```python
from build123d import *

# Parameters (mm, degrees)
BOSS_EXTRUDE1_DEPTH = 2
CUT_EXTRUDE1_REACH  = 137.359
SKETCH2_W           = 110
SKETCH2_H           = 10
SKETCH3_W           = 15
SKETCH3_H           = 4
BOSS_EXTRUDE2_DEPTH = 4


with BuildPart() as part:
    # Sketch1 → Boss-Extrude1 (new, symmetric)
    with BuildSketch(Plane.XY):
        Polygon((-105, -5), (-75, -5), (-75, -9), (-45, -9), (-45, -5), (-15, -5), (-15, -9), (15, -9), (15, -5), (45, -5), (45, -9), (75, -9), (75, -5), (105, -5), (105, -9), (135, -9), (135, -5), (135, 5), (135, 9), (105, 9), (105, 5), (75, 5), (75, 9), (45, 9), (45, 5), (15, 5), (15, 9), (-15, 9), (-15, 5), (-45, 5), (-45, 9), (-75, 9), (-75, 5), (-105, 5), (-105, 9), (-135, 9), (-135, 5), (-135, -5), (-135, -9), (-105, -9), align=None)
    extrude(amount=BOSS_EXTRUDE1_DEPTH, both=True)

    # Sketch2 → Cut-Extrude1 (cut, up to next)
    with BuildSketch(Plane.XY.offset(2), mode=Mode.PRIVATE) as cut_extrude1_sk1:
        with Locations((80, 4)):
            Rectangle(SKETCH2_W, SKETCH2_H)
    cut_extrude1_tool1 = extrude(cut_extrude1_sk1.sketch, amount=-CUT_EXTRUDE1_REACH, mode=Mode.PRIVATE) & part.part
    add(cut_extrude1_tool1.solids().sort_by_distance((80, 4, 2))[0], mode=Mode.SUBTRACT)

    # Sketch3 → Boss-Extrude2 (add)
    with BuildSketch(Plane.XY.offset(2)):
        with Locations((142.5, -3)):
            Rectangle(SKETCH3_W, SKETCH3_H)
    extrude(amount=-BOSS_EXTRUDE2_DEPTH)


solid = part.part
```
For this review, take the finished solid that the model builds, in its own axes (mm). Coordinates: 2 decimals unless noted, no trailing zeros. Write each loop counter-clockwise with the first axis right and the second up, starting at its lowest first coordinate (ties: lowest second). Pieces come first, ordered by that corner, then holes. Notation, with made-up numbers: (-9, 8.25) - (49, 8.25) arc R20 cw to (49, 46.25) - close; hole circle Ø10 at (25.25, 3.5). An arc over 180 degrees is marked (long way). Put each result on its own line as item: value.
1. Add section C-C, the plane x = 90.5. Give the boundary of the cut face in (y, z).
Values found:
outline: (-5, -2) - (-1, -2) - (-1, 2) - (-5, 2) - close
2. For pin 1 (1.2 mm diameter, centred on y = -7.5, z = 0.5, fed in from +X); pin 2 (2 mm diameter, centred on x = -93.5, z = -0.5, fed in from +Y); pin 3 (2 mm diameter, centred on x = -23.5, z = -1, fed in from -Y), all flat-tipped, find the tip position at first contact; note any pin that passes through.
Values found:
pin 1: x = 135
pin 2: y = 5
pin 3: y = -5
3. Add section B-B, the plane x = 54.5. Give the boundary of the cut face in (y, z).
Values found:
outline: (-9, -2) - (-1, -2) - (-1, 2) - (-9, 2) - close
4. Wall thickness on probe 1 along X at (y, z) = (-6, 1.5); probe 2 along X at (y, z) = (5.75, -0.2); probe 3 along X at (y, z) = (-0.5, -1.5): over which ranges is each line inside the solid? List them lowest first.
Values found:
probe 1: -135 to -105, -75 to -45, -15 to 15, 45 to 75, 105 to 135
probe 2: -135 to -105, -75 to -45, -15 to 15
probe 3: -135 to 25
